Work out the finished part from the listing and answer in its coordinate system (mm). A direction names the side the tool comes from. Coordinates: 2 decimals unless noted, no trailing zeros. Loops run counter-clockwise (first coordinate to the right, second up) from the corner with the lowest first, then second, coordinate; pieces in that order, holes last. Notation, with made-up numbers: (84, 0) - (122, 0) arc R10 cw to (122, 5) - close; hole circle Ø10 at (33.5, -38.5). An arc over 180 degrees is marked (long way). Write each question's results on one line, items separated by ' | '. Start each with the question number.
1. Determine the mould class of faces 6 (the flat face through (-0.25, 1, 1)), 7 (the flat face through (-1, 1, -0.25)), 8 (the cylindrical face through (-0.766, 0.542, 1.847)) for opening direction X: released by +X, released by -X, zero draft, split by the parting line, or undercut.
2. A cutting plane is placed at A-A on x = 0. Determine the outline of the cut face in (y, z).
3. Each of these flat-tipped pins is pushed along its axis until it touches: P1, Ø0.8, axis at y = 1, z = 1, coming from the -X side; P2, Ø0.5, axis at x = -1.5, y = 1, coming from the -Z side; P3, Ø0.5, axis at x = 1, y = 1, coming from the +Z side; P4, Ø1.8, axis at x = 0, z = 0, coming from the +Y side. Where does it stop, or does it pass through?
4. Find the intervals of material crossed by line 1 along X through (y, z) = (-8.25, 0.05); line 2 along Y through (x, z) = (0.1, -0.45); line 3 along Y through (x, z) = (1.2, -0.4), in increasing order. Write a range as [from, to].
5. A cutting plane is placed at B-B on z = 0. Determine the outline of the cut face in (x, y).
6. Which of the six approach directions +Z, -Z, +X, -X, +Y, -Y give full straight-line access (tool end or side, diameter ignored) to faces 1 (the flat face through (0.7, 1.6, -0.7)), 2 (the cylindrical face through (1, -6, 0)), 3 (the flat face through (0, 0.6, 0)), 4 (the flat face through (0.25, 1, -1)), 5 (the flat face through (1, 1, 0.25))?
7. A cutting plane is placed at C-C on y = -9. Determine the outline of the cut face in (x, z), then the cut area to 3 significant figures.
from build123d import *

# Parameters (mm, degrees)
SKETCH1_R           = 2
BOSS_EXTRUDE1_DEPTH = 1.6
FILLET1_R           = 0.5
SKETCH2_R           = 1
BOSS_EXTRUDE2_DEPTH = 12
CUT_EXTRUDE1_DEPTH  = 1


with BuildPart() as part:
    # Sketch1 → Boss-Extrude1 (new body)
    with BuildSketch(Plane(origin=(0, 0, 0), x_dir=(1, 0, 0), z_dir=(0, 1, 0))):
        with Locations(Location((0, 0, 0), (0, 0, 270))):
            Circle(SKETCH1_R)
    extrude(amount=BOSS_EXTRUDE1_DEPTH)

    # Fillet1
    fillet1_edges = [part.edges().sort_by_distance(p)[0] for p in [
        (0, 1.6, -2),
    ]]
    fillet(fillet1_edges, radius=FILLET1_R)

    # Sketch2 → Boss-Extrude2 (add)
    with BuildSketch(Plane.XZ):
        with Locations(Location((0, 0, 0), (0, 0, 90))):
            Circle(SKETCH2_R)
    extrude(amount=BOSS_EXTRUDE2_DEPTH)

    # Sketch3 → Cut-Extrude1 (cut)
    with BuildSketch(Plane(origin=(0, 1.6, 0), x_dir=(1, 0, 0), z_dir=(0, 1, 0))):
        with BuildLine():
            ThreePointArc((0.25, 1.479019946), (0, 1.5), (-0.25, 1.479019946))
            Line((-0.25, 1.479019946), (-0.25, 0.25))
            Line((-0.25, 0.25), (-1.479019946, 0.25))
            ThreePointArc((-1.479019946, 0.25), (-1.5, 0), (-1.479019946, -0.25))
            Line((-1.479019946, -0.25), (-0.25, -0.25))
            Line((-0.25, -0.25), (-0.25, -1.479019946))
            ThreePointArc((-0.25, -1.479019946), (0, -1.5), (0.25, -1.479019946))
            Line((0.25, -1.479019946), (0.25, -0.25))
            Line((0.25, -0.25), (1.479019946, -0.25))
            ThreePointArc((1.479019946, -0.25), (1.494745784, -0.12543939), (1.5, 0))
            ThreePointArc((1.5, 0), (1.494745784, 0.12543939), (1.479019946, 0.25))
            Line((1.479019946, 0.25), (0.25, 0.25))
            Line((0.25, 0.25), (0.25, 1.479019946))
        make_face()
        with BuildLine():
            Line((2, 0.25), (1.479019946, 0.25))
            ThreePointArc((1.479019946, 0.25), (1.494745784, 0.12543939), (1.5, 0))
            ThreePointArc((1.5, 0), (1.494745784, -0.12543939), (1.479019946, -0.25))
            Line((1.479019946, -0.25), (2, -0.25))
            Line((2, -0.25), (2, 0.25))
        make_face()
        with BuildLine():
            ThreePointArc((-1.479019946, -0.25), (-1.5, 0), (-1.479019946, 0.25))
            Line((-1.479019946, 0.25), (-2, 0.25))
            Line((-2, 0.25), (-2, -0.25))
            Line((-2, -0.25), (-1.479019946, -0.25))
        make_face()
        with BuildLine():
            Line((0.25, 2), (-0.25, 2))
            Line((-0.25, 2), (-0.25, 1.479019946))
            ThreePointArc((-0.25, 1.479019946), (0, 1.5), (0.25, 1.479019946))
            Line((0.25, 1.479019946), (0.25, 2))
        make_face()
    extrude(amount=-CUT_EXTRUDE1_DEPTH, mode=Mode.SUBTRACT)


solid = part.part
Values:
1) face 6: undercut | face 7: zero draft | face 8: split by the parting line
2) outline: (-12, -1) - (0, -1) - (0, -2) - (0.6, -2) - (0.6, 1.5) - (1.6, 1.5) arc R0.5 ccw to (1.1, 2) - (0, 2) - (0, 1) - (-12, 1) - close
3) P1: x = -1.91 | P2: z = -1.56 | P3: z = 1.85 | P4: y = 1.6
4) line 1: [-1, 1] | line 2: [-12, 0.6] | line 3: [0, 1.6]
5) outline: (-2, 0) - (-1, 0) - (-1, -12) - (1, -12) - (1, 0) - (2, 0) - (2, 0.6) - (-2, 0.6) - close
6) face 1: +Z, -Z, +X, -X, +Y | face 2: -Y | face 3: +Y | face 4: -Z, +Y | face 5: +X, -X, +Y
7) outline: circle Ø2 at (0, 0) | area: 3.14 mm^2
